Autodesk Inventor part; units mm, degrees
ref_plane "YZ Plane" through (0, 0, 0) normal (1, 0, 0) x (0, 1, 0)
ref_plane "XZ Plane" through (0, 0, 0) normal (0, 1, 0) x (-1, 0, 0)
ref_plane "XY Plane" through (0, 0, 0) normal (0, 0, 1) x (1, 0, 0)
sketch "Sketch9" plane through (0, 0, 0) normal (0, 1, 0) x (-1, 0, 0)
  line L0 (15, 15) -> (-15, 15)
  line L1 (-15, 15) -> (-15, -15)
  line L2 (-15, -15) -> (15, -15)
  line L3 (15, -15) -> (15, 15)
  line L4 (15, 15) -> (-15, -15) construction
  line L5 (-15, 15) -> (15, -15) construction
  line L6 (-13, 13) -> (13, 13)
  line L7 (13, 13) -> (13, -13)
  line L8 (13, -13) -> (-13, -13)
  line L9 (-13, -13) -> (-13, 13)
  point P0 (0, 0)
  dimension "d172" = 30
  dimension "d173" = 30
  dimension "d174" = 2
extrude "Extrusion3" add sketch "Sketch9" against normal blind 220
sketch "Sketch10" plane through (0, 0, 0) normal (1, 0, 0) x (0, 1, 0)
  line L0 (0, 15) -> (0, -15) construction
  line L1 (0, 15) -> (-220, 15) construction
  line L2 (-220, -15) -> (-220, 15) construction
  line L3 (0, -15) -> (-220, -15) construction
  line L4 (-201, 8.5) -> (-184, 8.5)
  line L5 (-184, 8.5) -> (-184, -8.5)
  line L6 (-184, -8.5) -> (-201, -8.5)
  line L7 (-201, -8.5) -> (-201, 8.5)
  line L8 (-201, 8.5) -> (-184, -8.5) construction
  line L9 (-184, 8.5) -> (-201, -8.5) construction
  circle A0 centre (-192.5, 0) radius 8.5
  line L10 (0, 15) -> (0, -15)
  point P0 (0, 0)
  point P1 (0, 0)
  point P2 (-220, 0)
  dimension "d177" = 17
  dimension "d178" = 17
  dimension "d191" = 19
extrude "Extrusion4" cut sketch "Sketch10" along normal through all contours A0
pattern_linear "Rectangular Pattern4" count 2 spacing 150 along (0, 1, 0) of "Extrusion4"
properties part number "ANP 1437 FDS WAY tube7" material "Stainless Steel"
Check sheet for the modelled part. Datum: model origin and axes. Units: mm. A direction names the side the tool comes from. Coordinates: 2 decimals unless noted, no trailing zeros. Write each loop counter-clockwise with the first axis right and the second up, starting at its lowest first coordinate (ties: lowest second). Pieces come first, ordered by that corner, then holes. Notation, with made-up numbers: M -7.5,21.25 L 9.5,21.25 A28 cw 9.5,47.25 Z; hole C 3.5,55 d2. An arc over 180 degrees is marked long. Use one line per item in the form item = value.
Item 1: Set-up check for faces 1 (the face through (13.986, -48.765, -5.745)), 2 (the face through (15, -108, 0)), 3 (the face through (-13, -108, 0)): record each of +Z, -Z, +X, -X, +Y, -Y from which the full face is reachable in a straight line by a thin tool's end or side.
Answer below:
face_1 = +X
face_2 = +Z, -Z, +X, +Y, -Y
face_3 = +Y, -Y
Item 2: Sectioned sample at D-D, the plane y = -178. Record the cut outline in (x, z).
Answer below:
outline = M -15,-15 L 15,-15 L 15,15 L -15,15 Z; hole M -13,-13 L 13,-13 L 13,13 L -13,13 Z
Item 3: Release check for a two-part mould opening along Y. For faces 4 (the face through (-15, -108, 0)), 5 (the face through (14, 0, 0)), 6 (the face through (14, -201, 0)) record: pulls with the +Y half, pulls with the -Y half, needs draft (parallel to the pull), parting line crosses it, or undercut.
Answer below:
face_4 = needs draft
face_5 = pulls with the +Y half
face_6 = undercut
Item 4: Sectioned sample at B-B, the plane z = 0. Record the cut outline in (x, y).
Answer below:
outline = M -15,-220 L -13,-220 L -13,0 L -15,0 Z; M 13,-220 L 15,-220 L 15,-201 L 13,-201 Z; M 13,-184 L 15,-184 L 15,-51 L 13,-51 Z; M 13,-34 L 15,-34 L 15,0 L 13,0 Z
Item 5: Gauge pin test, flat end, axial feed: pin 1 Ø2 at (y, z) = (-193, 1.5) entering from +X. Record the tip position at first contact, or that the pin passes through.
Answer below:
pin_1 = -13
Item 6: Sectioned sample at C-C, the plane x = -10. Record the cut outline in (y, z), and give its area (3 significant figures).
Answer below:
outline = M -220,-15 L 0,-15 L 0,-13 L -220,-13 Z; M -220,13 L 0,13 L 0,15 L -220,15 Z
area = 880 mm^2
Item 7: Material ranges on L1, parallel to Y at x = 14.1, z = 0; L2, parallel to X at y = -121, z = -8.25, recorded low to high. Write a range as from..to.
Answer below:
L1 = -220..-201, -184..-51, -34..0
L2 = -15..-13, 13..15
Item 8: Sectioned sample at A-A, the plane z = 10.75. Record the cut outline in (x, y).
Answer below:
outline = M -15,-220 L -13,-220 L -13,0 L -15,0 Z; M 13,-220 L 15,-220 L 15,0 L 13,0 Z
